```python
from build123d import *

# Parameters (mm, degrees)
SKETCH1_W           = 6
SKETCH1_H           = 2
BOSS_EXTRUDE2_DEPTH = 3
BOSS_EXTRUDE3_DEPTH = 2
CUT_EXTRUDE2_DEPTH  = 2
CUT_EXTRUDE3_DEPTH  = 1
BOSS_EXTRUDE5_DEPTH = 2
CUT_EXTRUDE4_DEPTH  = 1


with BuildPart() as part:
    # Sketch1 → Boss-Extrude2 (new body)
    with BuildSketch(Plane.XY):
        Rectangle(SKETCH1_W, SKETCH1_H)
    extrude(amount=BOSS_EXTRUDE2_DEPTH)

    # Sketch3 → Boss-Extrude3 (add)
    with BuildSketch(Plane(origin=(0, 0, 0), x_dir=(-1, 0, 0), z_dir=(0, 0, -1))):
        with BuildLine():
            Line((-2, 1), (3, 1))
            ThreePointArc((3, 1), (1.51763809, 2.931851653), (-0.732050808, 2))
            ThreePointArc((-0.732050808, 2), (-1.270020956, 1.378271238), (-2, 1))
        make_face()
    extrude(amount=-BOSS_EXTRUDE3_DEPTH)

    # Sketch4 → Cut-Extrude2 (cut)
    with BuildSketch(Plane.XY.offset(3)):
        with BuildLine():
            Line((0, -1), (0, 2.732050808))
            ThreePointArc((0, 2.732050808), (-1, 3), (-2, 2.732050808))
            Line((-2, 2.732050808), (-2, -1))
            Line((-2, -1), (0, -1))
        make_face()
    extrude(amount=-CUT_EXTRUDE2_DEPTH, mode=Mode.SUBTRACT)

    # Sketch5 → Cut-Extrude3 (cut)
    with BuildSketch(Plane.ZY):
        Polygon((2, 1), (3, 0), (3, 1), align=None)
    extrude(amount=-CUT_EXTRUDE3_DEPTH, mode=Mode.SUBTRACT)

    # Sketch6 → Boss-Extrude5 (add)
    with BuildSketch(Plane(origin=(0, 1, 0), x_dir=(1, 0, 0), z_dir=(0, 1, 0))):
        with BuildLine():
            ThreePointArc((-3, -4), (-1, -6), (1, -4))
            ThreePointArc((1, -4), (1.292893219, -3.292893219), (2, -3))
            Line((2, -3), (0, -3))
            Line((0, -3), (0, -4))
            ThreePointArc((0, -4), (-1, -5), (-2, -4))
            Line((-2, -4), (-2, -3))
            Line((-2, -3), (-3, -3))
            Line((-3, -3), (-3, -4))
        make_face()
    extrude(amount=-BOSS_EXTRUDE5_DEPTH)

    # Sketch7 → Cut-Extrude4 (cut)
    with BuildSketch(Plane(origin=(0, 1, 0), x_dir=(1, 0, 0), z_dir=(0, 1, 0))):
        with BuildLine():
            Line((-2, -4), (-3, -4))
            ThreePointArc((-3, -4), (-1, -6), (1, -4))
            ThreePointArc((1, -4), (1.292893219, -3.292893219), (2, -3))
            Line((2, -3), (0, -3))
            Line((0, -3), (0, -4))
            ThreePointArc((0, -4), (-1, -5), (-2, -4))
        make_face()
    extrude(amount=-CUT_EXTRUDE4_DEPTH, mode=Mode.SUBTRACT)


solid = part.part
```
Build history of the part. All positions in model axes, mm. A direction names the side the tool comes from. Round coordinates to 2 decimals unless told otherwise and drop trailing zeros. Write each loop counter-clockwise with the first axis right and the second up, starting at its lowest first coordinate (ties: lowest second). Pieces come first, ordered by that corner, then holes.
1) Band-saw the part on B-B, the plane z = 2.75. List the corners of the cut face in (x, y), and give its area (3 significant figures).
2) 3-axis set-ups, long thin cutter, end or side, ignore diameter. For faces 5 (the flat face through (-0.5, 0, 5.1)), 6 (the flat face through (-2.5, 1, 3)), 7 (the flat face through (1, 0.7, 2.7)): which of +Z, -Z, +X, -X, +Y, -Y reach the whole face in a straight line?
3) Drill centre lines: probe 1 along Z at (x, y) = (-2.1, 1.95); probe 2 along Z at (x, y) = (-0.45, 1); probe 3 along X at (y, z) = (0.7, 3.25). Where is each one in solid material? Low to high.
4) Band-saw the part on D-D, the plane z = 0.7. List the corners of the cut face in (x, y).
5) Pin check, flat tips, straight feed: pin 1 (0.9 mm diameter, centred on x = 0.5, y = 2, fed in from +Z); pin 2 (0.6 mm diameter, centred on x = 2, z = 1, fed in from +Y); pin 3 (0.5 mm diameter, centred on x = -2.5, y = 0.5, fed in from +Z). Stop position of each tip, or through.
6) Band-saw the part on C-C, the plane y = -0.15. List the corners of the cut face in (x, z).
7) Band-saw the part on A-A, the plane x = -1. List the corners of the cut face in (y, z).
8) Mould opens along X. For faces 1 (the flat face through (0.5, 0.5, 2.5)), 2 (the cylindrical face through (-1, -0.5, 6)), 3 (the flat face through (-1, 1, 1)), 4 (the flat face through (1, -1, 2)) say: +X half, -X half, draft (parallel to the pull), parting line (faces both ways), or undercut.
Ans:
1. outline: (-3, -1) - (-2, -1) - (-2, 1) - (-3, 1) - close; (0, -1) - (3, -1) - (3, 1) - (1, 1) - (1, 0.25) - (0, 0.25) - close
1. area: 7.25 mm2
2. face 5: +Z, +X, +Y
2. face 6: +Z, +X, -X, +Y
2. face 7: +Z, +Y
3. probe 1: z = 0 to 2
3. probe 2: z = 0 to 1
3. probe 3: x = -3 to -2
4. outline: (-3, -1) - (3, -1) - (3, 1) - (2, 1) arc R2.18 cw to (0.73, 2) arc R2 ccw to (-3, 1) - close
5. pin 1: stops at z = 2
5. pin 2: stops at y = 1.11
5. pin 3: stops at z = 4
6. outline: (-3, 0) - (3, 0) - (3, 3) - (2, 3) arc R1 cw to (1, 4) arc R2 ccw to (-3, 4) - close; hole (-2, 1) - (0, 1) - (0, 4) arc R1 ccw to (-2, 4) - close
7. outline: (-1, 0) - (3, 0) - (3, 1) - (-1, 1) - close; (-1, 5) - (0, 5) - (0, 6) - (-1, 6) - close
8. face 1: undercut
8. face 2: parting line
8. face 3: undercut
8. face 4: draft
